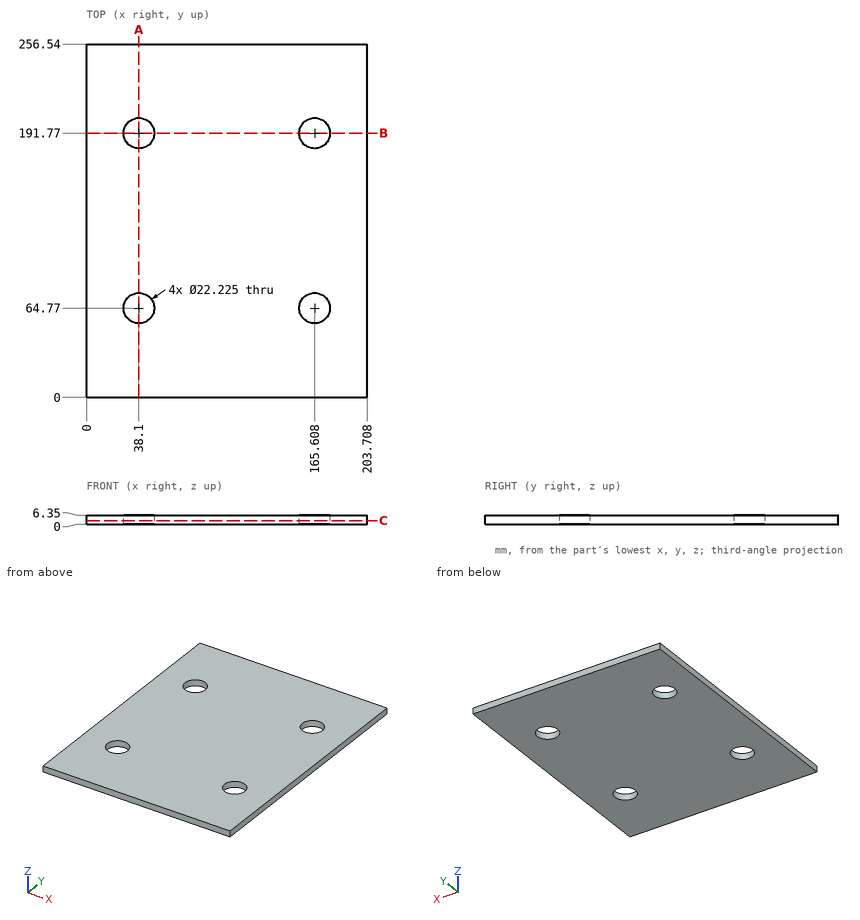
Job drawing, mm, ordinate dimensions from the low corner. One solid piece. Give positions to 0.01 mm unless a question says otherwise; leave off trailing zeros. Order: outer loops, then holes, each group sorted by start corner. A loop starts at its lowest first (then second) coordinate and runs counter-clockwise, first axis right, second up. Notation, with made-up numbers: (-14, 43) - (44, 43) arc R26 ccw to (44, 79) - close; hole circle Ø5 at (-20, 18.25). An arc over 180 degrees is marked (long way). Return JSON: item names as keys, results as strings.
1) Probe line 1 (Y direction, x = 38.1, z = 5); line 2 (Y direction, x = 161.5, z = 5.5); line 3 (X direction, y = 56, z = 1.5). List the from-to ranges inside material, lowest first. Write a range as from..to.
Geometry says:
{"line 1": "0..53.66, 75.88..180.66, 202.88..256.54", "line 2": "0..54.44, 75.1..181.44, 202.1..256.54", "line 3": "0..31.28, 44.92..158.78, 172.43..203.71"}
2) Cut at C-C, the plane z = 2.5. Give the cut face in (x, y) (1 decimal), plus the area to 3 significant figures.
Geometry says:
{"outline": "(0, 0) - (203.7, 0) - (203.7, 256.5) - (0, 256.5) - close; hole circle Ø22.2 at (38.1, 64.8); hole circle Ø22.2 at (38.1, 191.8); hole circle Ø22.2 at (165.6, 64.8); hole circle Ø22.2 at (165.6, 191.8)", "area": "50,700 mm²"}
3) Cut at B-B, the plane y = 191.77. Give the cut face in (x, z).
Geometry says:
{"outline": "(0, 0) - (26.99, 0) - (26.99, 6.35) - (0, 6.35) - close; (49.21, 0) - (154.5, 0) - (154.5, 6.35) - (49.21, 6.35) - close; (176.72, 0) - (203.71, 0) - (203.71, 6.35) - (176.72, 6.35) - close"}
4) Cut at A-A, the plane x = 38.1. Give the cut face in (y, z).
Geometry says:
{"outline": "(0, 0) - (53.66, 0) - (53.66, 6.35) - (0, 6.35) - close; (75.88, 0) - (180.66, 0) - (180.66, 6.35) - (75.88, 6.35) - close; (202.88, 0) - (256.54, 0) - (256.54, 6.35) - (202.88, 6.35) - close"}
5) Flat gauge pin, fed straight in: P1, Ø18, axis at x = 165.608, y = 64.77, coming from the +Z side. Where does the tip first touch, or does it go through?
Geometry says:
{"P1": "through"}
